Work out the finished part from the listing and answer in its coordinate system (mm). Face numbers are marked on the shaded views. A direction names the side the tool comes from. Round coordinates to 2 decimals unless told otherwise and drop trailing zeros. Order: outer loops, then holes, each group sorted by start corner. A loop starts at its lowest first (then second) coordinate and runs counter-clockwise, first axis right, second up. Notation, with made-up numbers: (-11, 18.5) -> (7, 18.5) arc R23 ccw to (7, 44.5) -> close; hole circle Ø6 at (56.25, 77). An arc over 180 degrees is marked (long way). Use one line per item in the form item = value.
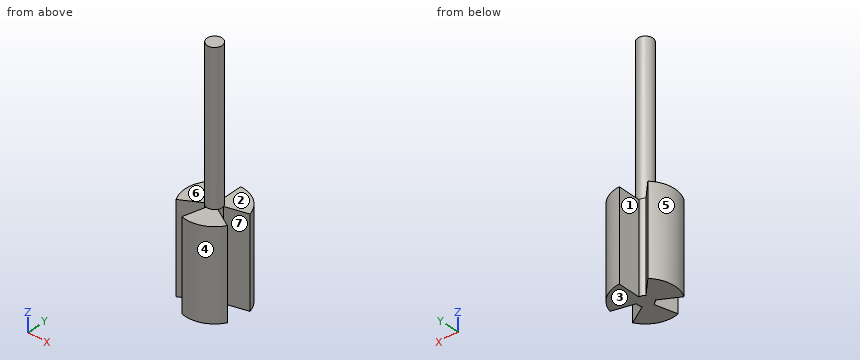
```python
from build123d import *

# Parameters (mm, degrees)
SKETCH1_R           = 251.46
BOSS_EXTRUDE1_DEPTH = 762
CUT_EXTRUDE1_DEPTH  = 841.897296464
BOSS_EXTRUDE2_START = 1270
SKETCH3_R           = 63.5
BOSS_EXTRUDE2_DEPTH = 1270


with BuildPart() as part:
    # Sketch1 → Boss-Extrude1 (new body)
    with BuildSketch(Plane.XY):
        Circle(SKETCH1_R)
    extrude(amount=BOSS_EXTRUDE1_DEPTH)

    # Sketch2 → Cut-Extrude1 (cut, through all)
    with BuildSketch(Plane.XY.offset(762)):
        with BuildLine():
            Line((-44.901280605, 44.901280605), (-177.809071197, 177.809071197))
            ThreePointArc((-177.809071197, 177.809071197), (-96.229575903, 232.318747245), (0, 251.46))
            Line((0, 251.46), (0, 63.5))
            ThreePointArc((0, 63.5), (-24.300397955, 58.666350314), (-44.901280605, 44.901280605))
        make_face()
        with BuildLine():
            Line((61.336289969, 16.435009364), (242.891708279, 65.082637081))
            ThreePointArc((242.891708279, 65.082637081), (249.308724841, -32.822116296), (217.770748036, -125.73))
            Line((217.770748036, -125.73), (54.99261314, -31.75))
            ThreePointArc((54.99261314, -31.75), (62.956748697, -8.288413206), (61.336289969, 16.435009364))
        make_face()
        with BuildLine():
            Line((-16.435009364, -61.336289969), (-65.082637081, -242.891708279))
            ThreePointArc((-65.082637081, -242.891708279), (-153.079148939, -199.49663095), (-217.770748036, -125.73))
            Line((-217.770748036, -125.73), (-54.99261314, -31.75))
            ThreePointArc((-54.99261314, -31.75), (-38.656350742, -50.377937108), (-16.435009364, -61.336289969))
        make_face()
    extrude(amount=-CUT_EXTRUDE1_DEPTH, mode=Mode.SUBTRACT)

    # Sketch3 → Boss-Extrude2 (add)
    with BuildSketch(Plane.XY.offset(762).offset(BOSS_EXTRUDE2_START)):
        Circle(SKETCH3_R)
    extrude(amount=-BOSS_EXTRUDE2_DEPTH)


solid = part.part
```
Item 1: Determine the mould class of the marked faces 4, 5, 6 and 7 for opening direction Y: released by +Y, released by -Y, zero draft, split by the parting line, or undercut.
Findings:
face_4 = released by -Y
face_5 = split by the parting line
face_6 = zero draft
face_7 = undercut
Item 2: The part is cut by section B-B, the plane x = 158. Give the vertices of the cut face in (y, z).
Findings:
outline = (-195.62, 0) -> (-91.22, 0) -> (-91.22, 762) -> (-195.62, 762) -> close; (42.34, 0) -> (195.62, 0) -> (195.62, 762) -> (42.34, 762) -> close
Item 3: The part is cut by section D-D, the plane x = -147.5. Give the vertices of the cut face in (y, z), and give its area (3 significant figures).
Findings:
outline = (-85.16, 0) -> (147.5, 0) -> (147.5, 762) -> (-85.16, 762) -> close
area = 177,000 mm^2
Item 4: Flat-ended cylindrical pins translate along their axes: P1, Ø12, axis at x = -139.5, y = 85.5, coming from the +Z side; P2, Ø4, axis at x = -16.5, z = 648.5, coming from the -Y side; P3, Ø3, axis at y = -46.5, z = 1537.5, coming from the -X side. Find the tip coordinate at first contact, or state that the pin passes through.
Findings:
P1 = 762
P2 = -251.04
P3 = -44.8
Item 5: Consider line 1 along Z through (x, y) = (-142.5, 112.5); line 2 along X through (y, z) = (81.5, 137.5); line 3 along X through (y, z) = (-125, 323.5). Determine where each line is inside the solid, lowest interval first.
Findings:
line_1 = 0 to 762
line_2 = -237.89 to -81.5, 0 to 237.89
line_3 = -218.19 to -216.51, -33.49 to 216.51
Item 6: The part is cut by section C-C, the plane y = -181.5. Give the vertices of the cut face in (x, z), and give its area (3 significant figures).
Findings:
outline = (-48.63, 0) -> (174.04, 0) -> (174.04, 762) -> (-48.63, 762) -> close
area = 170,000 mm^2
Item 7: For the marked faces 1, 2 and 3, determine the directions among +Z, -Z, +X, -X, +Y, -Y from which every point of the face is accessible in a straight line to the end or side of a thin tool.
Findings:
face_1 = +Z, -Z, +Y
face_2 = +Z, +X, +Y
face_3 = -Z, +X, -X, +Y, -Y
Item 8: The part is cut by section A-A, the plane z = 726. Give the vertices of the cut face in (x, y) (3 decimals).
Findings:
outline = (-217.771, -125.73) -> (-54.993, -31.75) arc R63.5 ccw to (-16.435, -61.336) -> (-65.083, -242.892) arc R251.46 ccw to (217.771, -125.73) -> (54.993, -31.75) arc R63.5 ccw to (61.336, 16.435) -> (242.892, 65.083) arc R251.46 ccw to (0, 251.46) -> (0, 63.5) arc R63.5 ccw to (-44.901, 44.901) -> (-177.809, 177.809) arc R251.46 ccw to start
